```python
from build123d import *

# Parameters (mm, degrees)
ESQUISSE1_W             = 300
ESQUISSE1_H             = 130
BOSS_EXTRU_2_DEPTH      = 130
ESQUISSE6_W             = 280
ESQUISSE6_H             = 110
ENL_V_MAT_EXTRU_1_DEPTH = 120
CONG_2_R                = 1
CONG_3_R                = 1
CONG_4_R                = 1
CONG_5_R                = 1
CONG_6_R                = 1
CONG_7_R                = 1
ESQUISSE7_R             = 4
ENL_V_MAT_EXTRU_2_DEPTH = 257.497602135


with BuildPart() as part:
    # Esquisse1 → Boss.-Extru.2 (new body)
    with BuildSketch(Plane.XY):
        with Locations((35.717581023, 65)):
            Rectangle(ESQUISSE1_W, ESQUISSE1_H)
    extrude(amount=BOSS_EXTRU_2_DEPTH)

    # Esquisse6 → Enlèv. mat.-Extru.1 (cut)
    with BuildSketch(Plane(origin=(0, 130, 0), x_dir=(1, 0, 0), z_dir=(0, 1, 0))):
        with Locations((35.717581023, -65)):
            Rectangle(ESQUISSE6_W, ESQUISSE6_H)
    extrude(amount=-ENL_V_MAT_EXTRU_1_DEPTH, mode=Mode.SUBTRACT)

    # Congé2
    cong_2_edges = [part.edges().sort_by_distance(p)[0] for p in [
        (-104.282418977, 130, 65),
        (35.717581023, 130, 10),
    ]]
    fillet(cong_2_edges, radius=CONG_2_R)

    # Congé3
    cong_3_edges = [part.edges().sort_by_distance(p)[0] for p in [
        (35.217581023, 130, 120),
    ]]
    fillet(cong_3_edges, radius=CONG_3_R)

    # Congé4
    cong_4_edges = [part.edges().sort_by_distance(p)[0] for p in [
        (175.717581023, 130, 65),
    ]]
    fillet(cong_4_edges, radius=CONG_4_R)

    # Congé5
    cong_5_edges = [part.edges().sort_by_distance(p)[0] for p in [
        (35.717581023, 130, 0),
        (-114.282418977, 130, 65),
    ]]
    fillet(cong_5_edges, radius=CONG_5_R)

    # Congé6
    cong_6_edges = [part.edges().sort_by_distance(p)[0] for p in [
        (36.217581023, 130, 130),
        (-114.282418977, 64.5, 130),
        (-113.989525758, 129.707106781, 130),
    ]]
    fillet(cong_6_edges, radius=CONG_6_R)

    # Congé7
    cong_7_edges = [part.edges().sort_by_distance(p)[0] for p in [
        (185.717581023, 64.5, 130),
        (185.717581023, 64.5, 0),
        (185.717581023, 129.707106781, 0.292893219),
        (185.717581023, 130, 65),
        (185.717581023, 129.707106781, 129.707106781),
    ]]
    fillet(cong_7_edges, radius=CONG_7_R)

    # Esquisse7 → Enlèv. mat.-Extru.2 (cut, through all)
    with BuildSketch(Plane.XY.offset(10)):
        with Locations((5.872475368, 119)):
            Circle(ESQUISSE7_R)
        with Locations((35.872475344, 119.001199684)):
            Circle(ESQUISSE7_R)
    extrude(amount=-ENL_V_MAT_EXTRU_2_DEPTH, mode=Mode.SUBTRACT)


solid = part.part
```
Verification items for the finished model (mm, model axes). A direction names the side the tool comes from. Give positions to 0.01 mm unless a question says otherwise; leave off trailing zeros. Write each loop counter-clockwise with the first axis right and the second up, starting at its lowest first coordinate (ties: lowest second). Pieces come first, ordered by that corner, then holes. Notation, with made-up numbers: M 9.25,36 L 14.25,36 A19 cw 14.25,61 Z; hole C -27.75,-32.5 d10. An arc over 180 degrees is marked long. One line per question, with ' | ' between items.
1) Thickness scan on line 1 along Z through (x, y) = (-52, 75.5); line 2 along X through (y, z) = (35.5, 112); line 3 along Y through (x, z) = (122, 16). Record the ranges inside material, lowest first. Write a range as [from, to].
Result:
line 1: z = [0, 10], [120, 130] | line 2: x = [-114.28, -104.28], [175.72, 185.72] | line 3: y = [0, 10]
2) Mould release check, pull along Z, two halves, no side actions. Record for faces 4 (the flat face through (34, 65, 130)), 5 (the flat face through (175.718, 70, 66)), 6 (the flat face through (34, 70, 120)), 7 (the flat face through (-114.282, 64, 64)): released by +Z, released by -Z, zero draft, split by the parting line, or undercut.
Result:
face 4: released by +Z | face 5: undercut | face 6: undercut | face 7: zero draft
3) Section check B-B on y = 22. Enter the section's corners in (x, z), plus the area to 3 significant figures.
Result:
outline: M -114.28,0 L 184.72,0 A1 ccw 185.72,1 L 185.72,129 A1 ccw 184.72,130 L -113.28,130 A1 ccw -114.28,129 Z; hole M -104.28,10 L 175.72,10 L 175.72,120 L -104.28,120 Z | area: 8,200 mm2
4) Gauge pin test, flat end, axial feed: pin 1 Ø6 at (x, z) = (-56.5, 55) entering from +Y. Record the tip position at first contact, or that the pin passes through.
Result:
pin 1: stops at y = 10
5) Section check A-A on x = -78. Enter the section's corners in (y, z).
Result:
outline: M 0,0 L 129,0 A1 ccw 130,1 L 130,9 A1 ccw 129,10 L 10,10 L 10,120 L 129,120 A1 ccw 130,121 L 130,129 A1 ccw 129,130 L 0,130 Z
6) Set-up check for faces 1 (the cylindrical face through (5.352, 122.966, 5.07)), 2 (the flat face through (-104.282, 70, 66)), 3 (the flat face through (34, 0, 64)): record each of +Z, -Z, +X, -X, +Y, -Y from which the full face is reachable in a straight line by a thin tool's end or side.
Result:
face 1: -Z | face 2: +Y | face 3: +Z, -Z, +X, -X, -Y
7) Section check C-C on z = 59.5. Enter the section's corners in (x, y).
Result:
outline: M -114.28,0 L 185.72,0 L 185.72,129 A1 ccw 184.72,130 L 176.72,130 A1 ccw 175.72,129 L 175.72,10 L -104.28,10 L -104.28,129 A1 ccw -105.28,130 L -113.28,130 A1 ccw -114.28,129 Z
